Can you work these out from the drawing? Everything is in mm from the part's minimum corner. A direction names the side the tool comes from. Round coordinates to 2 decimals unless told otherwise and drop trailing zeros. Write each loop counter-clockwise with the first axis right and the second up, starting at its lowest first coordinate (ties: lowest second). Pieces come first, ordered by that corner, then holes. Notation, with made-up numbers: M 24,-30.5 L 73,-30.5 A24 ccw 73,-6.5 Z; hole C -28.75,-16 d10. An arc over 180 degrees is marked long. Answer in a Markdown table with one row per item. Add a question column.
(1) Suppose I cut it at A-A, the plane z = 46. Write out the boundary of the cut face in (x, y).
(2) If we mould it in two halves opening along Y, with no side actions, what happens to the marked faces 1, 2, 3 and 4? For each: released by +Y, released by -Y, zero draft, split by the parting line, or undercut.
(3) For the marked faces 5, 6 and 7, which set-ups out of +Z, -Z, +X, -X, +Y, -Y let a thin tool reach every point of the face, with its end or its side?
(4) I'm going to push flat-ended pins straight in: pin 1 (8 mm diameter, centred on y = 16, z = 46, fed in from -X); pin 2 (15 mm diameter, centred on y = 16, z = 46, fed in from +X); pin 3 (16 mm diameter, centred on y = 11.5, z = 27.5, fed in from -X); pin 4 (7.5 mm diameter, centred on x = 9, y = 15.5, fed in from +Z). Where does each tip first touch, or does it pass through?
(5) Suppose I cut it at D-D, the plane z = 54. Write out the boundary of the cut face in (x, y), then the cut area to 3 significant figures.
(6) Suppose I cut it at C-C, the plane y = 30. Write out the boundary of the cut face in (x, z), then the cut area to 3 significant figures.
(7) If I drill on probe 1 along Y at (x, z) = (12.5, 9.5); probe 2 along Z at (x, y) = (39.5, 16); probe 3 along X at (y, z) = (23.5, 45), over which ranges is the centre line in solid material (lowest first)?
(8) Suppose I cut it at B-B, the plane x = 100. Write out the boundary of the cut face in (y, z).
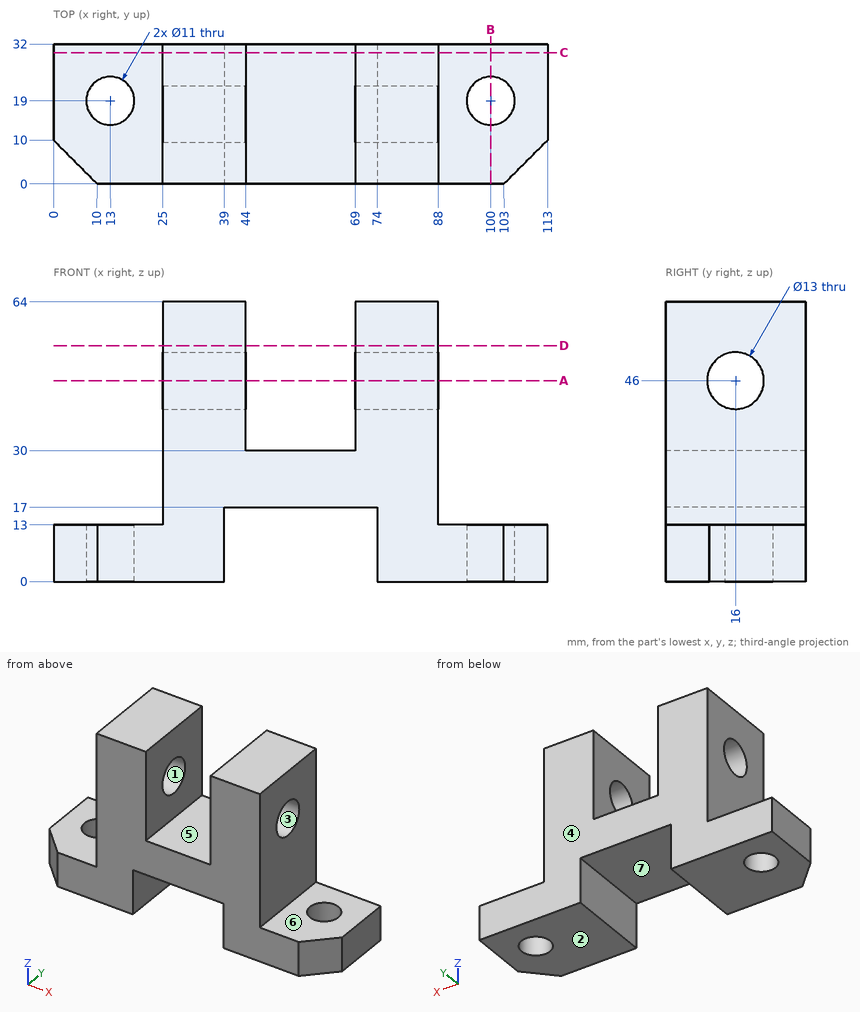
Calculated:
| question | item | result |
|---|---|---|
| 1 | outline | M 25,0 L 44,0 L 44,9.5 L 25,9.5 Z; M 25,22.5 L 44,22.5 L 44,32 L 25,32 Z; M 69,0 L 88,0 L 88,9.5 L 69,9.5 Z; M 69,22.5 L 88,22.5 L 88,32 L 69,32 Z |
| 2 | face 1 | undercut |
| 2 | face 2 | zero draft |
| 2 | face 3 | undercut |
| 2 | face 4 | released by +Y |
| 3 | face 5 | +Z, +Y, -Y |
| 3 | face 6 | +Z, +X, +Y, -Y |
| 3 | face 7 | -Z, +Y, -Y |
| 4 | pin 1 | through |
| 4 | pin 2 | x = 88 |
| 4 | pin 3 | x = 25 |
| 4 | pin 4 | z = 13 |
| 5 | outline | M 25,0 L 44,0 L 44,32 L 25,32 Z; M 69,0 L 88,0 L 88,32 L 69,32 Z |
| 5 | area | 1,220 mm² |
| 6 | outline | M 0,0 L 39,0 L 39,17 L 74,17 L 74,0 L 113,0 L 113,13 L 88,13 L 88,64 L 69,64 L 69,30 L 44,30 L 44,64 L 25,64 L 25,13 L 0,13 Z |
| 6 | area | 3,240 mm² |
| 7 | probe 1 | 0 to 13.52, 24.48 to 32 |
| 7 | probe 2 | 17 to 39.5, 52.5 to 64 |
| 7 | probe 3 | 25 to 44, 69 to 88 |
| 8 | outline | M 0,0 L 13.5,0 L 13.5,13 L 0,13 Z; M 24.5,0 L 32,0 L 32,13 L 24.5,13 Z |
